Verification items for the finished model (mm, model axes). Round coordinates to 2 decimals unless told otherwise and drop trailing zeros. Write each loop counter-clockwise with the first axis right and the second up, starting at its lowest first coordinate (ties: lowest second). Pieces come first, ordered by that corner, then holes. Notation, with made-up numbers: M -27.5,37 L 16.5,37 A16 cw 16.5,64 Z; hole C 64,68 d5. An arc over 180 degrees is marked long. One line per item, written item: value. Start each with the question number.
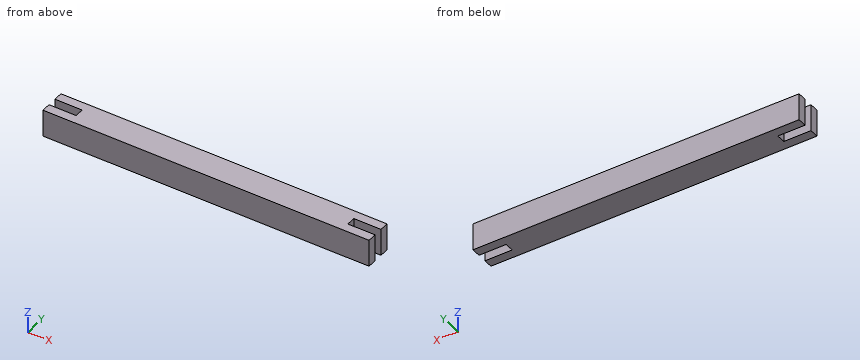
from build123d import *

# Parameters (mm, degrees)
CROQUIS1_W              = 300
CROQUIS1_H              = 30
SALIENTE_EXTRUIR1_DEPTH = 15
SALIENTE_EXTRUIR2_START = 10
CROQUIS2_W              = 360
CROQUIS2_H              = 30
SALIENTE_EXTRUIR2_DEPTH = 5


with BuildPart() as part:
    # Croquis1 → Saliente-Extruir1 (new, symmetric)
    with BuildSketch(Plane(origin=(0, 0, 0), x_dir=(1, 0, 0), z_dir=(0, 1, 0))):
        with Locations((0, 215)):
            Rectangle(CROQUIS1_W, CROQUIS1_H)
    extrude(amount=SALIENTE_EXTRUIR1_DEPTH, both=True)

    # Croquis2 → Saliente-Extruir2 (add, symmetric)
    with BuildSketch(Plane(origin=(0, 0, 0), x_dir=(1, 0, 0), z_dir=(0, 1, 0)).offset(SALIENTE_EXTRUIR2_START)):
        with Locations((0, 215)):
            Rectangle(CROQUIS2_W, CROQUIS2_H)
    saliente_extruir2 = extrude(amount=SALIENTE_EXTRUIR2_DEPTH, both=True)

    # Simetría1: Saliente-Extruir2 across plane
    add(saliente_extruir2.mirror(Plane.ZX))


solid = part.part
1) Cross-section at B-B (y = 0.5). Record the boundary of the cut face in (x, z), then the cut area to 3 significant figures.
2) Gauge pin test, flat ends, axial feed: pin 1 Ø3 at (y, z) = (3, -208) entering from +X; pin 2 Ø4 at (y, z) = (2, -219.5) entering from -X. Record the tip position at first contact, or that the pin passes through.
3) Cross-section at A-A (z = -204.25). Record the boundary of the cut face in (x, y), then the cut area to 3 significant figures.
4) Thickness scan on line 1 (Y direction, x = -161, z = -215.5); line 2 (X direction, y = -4.5, z = -201.75). Record the ranges inside material, lowest first.
Results below:
1. outline: M -150,-230 L 150,-230 L 150,-200 L -150,-200 Z
1. area: 9,000 mm²
2. pin 1: stops at x = 150
2. pin 2: stops at x = -150
3. outline: M -180,-15 L 180,-15 L 180,-5 L 150,-5 L 150,5 L 180,5 L 180,15 L -180,15 L -180,5 L -150,5 L -150,-5 L -180,-5 Z
3. area: 10,200 mm²
4. line 1: y = -15 to -5, 5 to 15
4. line 2: x = -150 to 150
